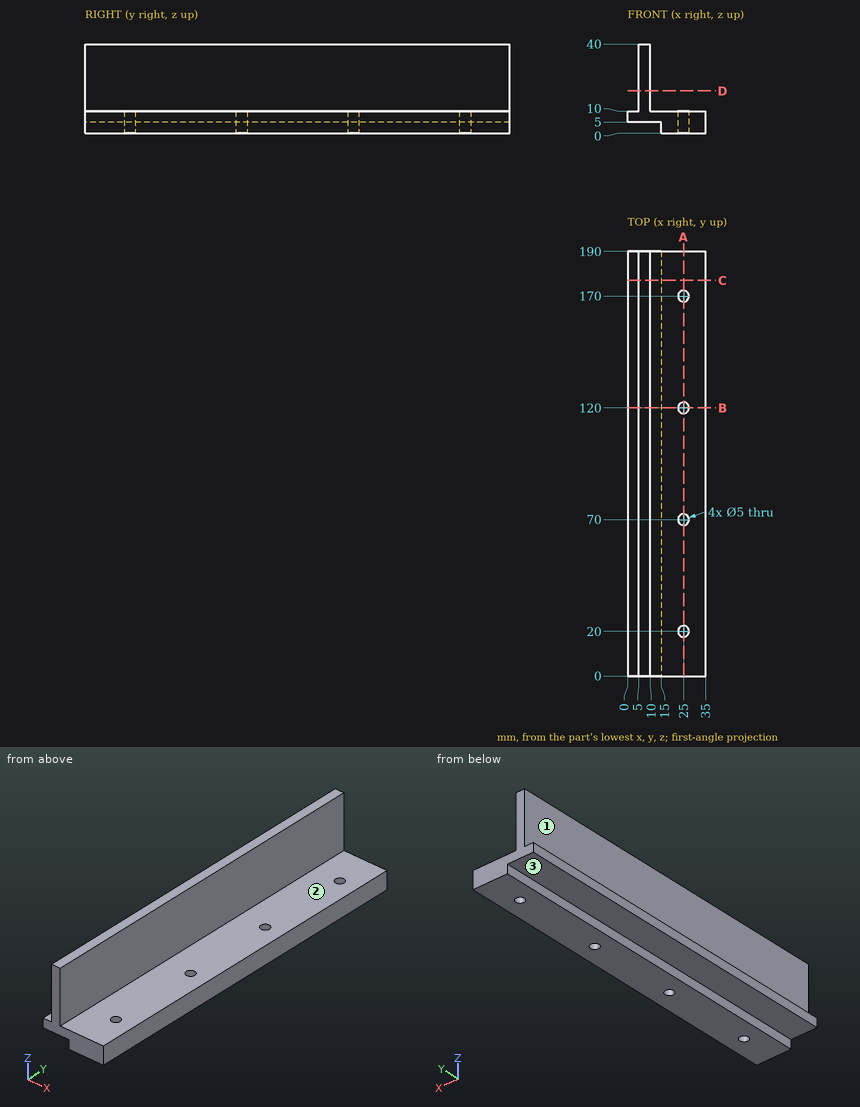
Job drawing, mm, ordinate dimensions from the low corner. One solid piece. A direction names the side the tool comes from. Round coordinates to 2 decimals unless told otherwise and drop trailing zeros. Write each loop counter-clockwise with the first axis right and the second up, starting at its lowest first coordinate (ties: lowest second). Pieces come first, ordered by that corner, then holes.
1) Band-saw the part on B-B, the plane y = 120. List the corners of the cut face in (x, z), and give its area (3 significant figures).
2) Drill centre lines: probe 1 along Y at (x, z) = (25, 4); probe 2 along Y at (x, z) = (23, 5); probe 3 along Z at (x, y) = (18, 14). Where is each one in solid material? Low to high.
3) 3-axis set-ups, long thin cutter, end or side, ignore diameter. For the marked faces 1, 2 and 3: which of +Z, -Z, +X, -X, +Y, -Y reach the whole face in a straight line?
4) Band-saw the part on C-C, the plane y = 177. List the corners of the cut face in (x, z), and give its area (3 significant figures).
5) Pin check, flat tips, straight feed: pin 1 (6 mm diameter, centred on x = 20, y = 24.5, fed in from +Z); pin 2 (15 mm diameter, centred on y = 122, z = 26, fed in from -X); pin 3 (7.5 mm diameter, centred on x = 4, y = 50, fed in from -Z). Stop position of each tip, or through.
6) Band-saw the part on A-A, the plane x = 25. List the corners of the cut face in (y, z), and give its area (3 significant figures).
7) Band-saw the part on D-D, the plane z = 19. List the corners of the cut face in (x, y).
Ans:
1. outline: (0, 5) - (15, 5) - (15, 0) - (22.5, 0) - (22.5, 10) - (10, 10) - (10, 40) - (5, 40) - (5, 10) - (0, 10) - close; (27.5, 0) - (35, 0) - (35, 10) - (27.5, 10) - close
1. area: 375 mm2
2. probe 1: y = 0 to 17.5, 22.5 to 67.5, 72.5 to 117.5, 122.5 to 167.5, 172.5 to 190
2. probe 2: y = 0 to 18.5, 21.5 to 68.5, 71.5 to 118.5, 121.5 to 168.5, 171.5 to 190
2. probe 3: z = 0 to 10
3. face 1: +Z, -X, +Y, -Y
3. face 2: +Z, +X, +Y, -Y
3. face 3: -Z, -X, +Y, -Y
4. outline: (0, 5) - (15, 5) - (15, 0) - (35, 0) - (35, 10) - (10, 10) - (10, 40) - (5, 40) - (5, 10) - (0, 10) - close
4. area: 425 mm2
5. pin 1: stops at z = 10
5. pin 2: stops at x = 5
5. pin 3: stops at z = 5
6. outline: (0, 0) - (17.5, 0) - (17.5, 10) - (0, 10) - close; (22.5, 0) - (67.5, 0) - (67.5, 10) - (22.5, 10) - close; (72.5, 0) - (117.5, 0) - (117.5, 10) - (72.5, 10) - close; (122.5, 0) - (167.5, 0) - (167.5, 10) - (122.5, 10) - close; (172.5, 0) - (190, 0) - (190, 10) - (172.5, 10) - close
6. area: 1,700 mm2
7. outline: (5, 0) - (10, 0) - (10, 190) - (5, 190) - close
